```python
from build123d import *

# Parameters (mm, degrees)
SKETCH1_W           = 200
SKETCH1_H           = 150
BOSS_EXTRUDE1_DEPTH = 150
SKETCH2_R           = 14.834241456
CUT_EXTRUDE1_DEPTH  = 5
LPATTERN1_COUNT     = 3
LPATTERN1_PITCH     = 50
SKETCH3_W           = 17.49362466
SKETCH3_H           = 150
BOSS_EXTRUDE2_DEPTH = 50
SKETCH4_R           = 20.657727603
BOSS_EXTRUDE3_DEPTH = 30
SKETCH5_R           = 10
BOSS_EXTRUDE4_DEPTH = 60
SKETCH6_W           = 19.92759369
SKETCH6_H           = 8.419652836
SKETCH6_W_2         = 21.376212584
SKETCH6_H_2         = 8.0068992
CUT_EXTRUDE2_DEPTH  = 15


with BuildPart() as part:
    # Sketch1 → Boss-Extrude1 (new body)
    with BuildSketch(Plane.XY):
        Rectangle(SKETCH1_W, SKETCH1_H)
    extrude(amount=BOSS_EXTRUDE1_DEPTH)

    # Sketch2 → Cut-Extrude1 (cut)
    with BuildSketch(Plane(origin=(0, 0, 0), x_dir=(-1, 0, 0), z_dir=(0, 0, -1))):
        with Locations((80.018238541, 54.109118562)):
            Circle(SKETCH2_R)
    cut_extrude1 = extrude(amount=-CUT_EXTRUDE1_DEPTH, mode=Mode.SUBTRACT)

    # LPattern1: Cut-Extrude1 ×3
    with Locations(*[(0, -i * LPATTERN1_PITCH, 0) for i in range(1, LPATTERN1_COUNT)]):
        add(cut_extrude1, mode=Mode.SUBTRACT)

    # Sketch3 → Boss-Extrude2 (add)
    with BuildSketch(Plane(origin=(100, 0, 0), x_dir=(0, 0, -1), z_dir=(1, 0, 0))):
        with Locations((-125.713599326, 0)):
            Rectangle(SKETCH3_W, SKETCH3_H)
    extrude(amount=BOSS_EXTRUDE2_DEPTH)

    # Sketch4 → Boss-Extrude3 (add)
    with BuildSketch(Plane(origin=(0, 0, 116.966786996), x_dir=(-1, 0, 0), z_dir=(0, 0, -1))):
        with Locations(Location((-127.668059081, 0, 0), (0, 0, 180))):
            Circle(SKETCH4_R)
    extrude(amount=BOSS_EXTRUDE3_DEPTH)

    # Sketch5 → Boss-Extrude4 (add)
    with BuildSketch(Plane.XY.offset(150)):
        with Locations(Location((0, 0, 0), (0, 0, 180))):
            Circle(SKETCH5_R)
    extrude(amount=BOSS_EXTRUDE4_DEPTH)

    # Sketch6 → Cut-Extrude2 (cut)
    with BuildSketch(Plane.XY.offset(210)):
        with Locations((0.233720093, 6.517553958)):
            Rectangle(SKETCH6_W, SKETCH6_H)
        with Locations((-0.888741557, -5.9965504)):
            Rectangle(SKETCH6_W_2, SKETCH6_H_2)
    extrude(amount=-CUT_EXTRUDE2_DEPTH, mode=Mode.SUBTRACT)


solid = part.part
```
Build history of the part. All positions in model axes, mm. A direction names the side the tool comes from. Round coordinates to 2 decimals unless told otherwise and drop trailing zeros. Write each loop counter-clockwise with the first axis right and the second up, starting at its lowest first coordinate (ties: lowest second). Pieces come first, ordered by that corner, then holes.
1) Band-saw the part on A-A, the plane z = 97.5. List the corners of the cut face in (x, y).
2) Drill centre lines: probe 1 along X at (y, z) = (-32.5, 107.5); probe 2 along Z at (x, y) = (29, 11); probe 3 along Z at (x, y) = (102.5, 1). Where is each one in solid material? Low to high.
3) Pin check, flat tips, straight feed: pin 1 (12 mm diameter, centred on x = 4, z = 202, fed in from +Y); pin 2 (2.5 mm diameter, centred on x = 4.5, y = 5, fed in from +Z); pin 3 (9 mm diameter, centred on x = -75, y = -45.5, fed in from -Z); pin 4 (17 mm diameter, centred on y = 35, z = 140, fed in from +X). Stop position of each tip, or through.
4) Band-saw the part on C-C, the plane y = -42. List the corners of the cut face in (x, z), and give its area (3 significant figures).
5) Band-saw the part on B-B, the plane x = 0. List the corners of the cut face in (y, z).
6) Mould opens along X. For faces 6 (the flat face through (100, -1, 142)), 7 (the cylindrical face through (10, 0, 173)), 8 (the flat face through (0, 5, 195)), 9 (the cylindrical face through (-86.863, 40.949, 2.465)) say: +X half, -X half, draft (parallel to the pull), parting line (faces both ways), or undercut.
7) Band-saw the part on D-D, the plane z = 189.5. List the corners of the cut face in (x, y).
8) 3-axis set-ups, long thin cutter, end or side, ignore diameter. For faces 1 (the flat face through (-80, 4, 5)), 2 (the flat face through (125, -1, 134.46)), 3 (the flat face through (-1, 1, 0)), 4 (the flat face through (0, 2.308, 203)), 5 (the flat face through (0, -5, 195)): which of +Z, -Z, +X, -X, +Y, -Y reach the whole face in a straight line?
Ans:
1. outline: (-100, -75) - (100, -75) - (100, 75) - (-100, 75) - close; circle Ø41.32 at (127.67, 0)
2. probe 1: x = -100 to 100
2. probe 2: z = 0 to 150
2. probe 3: z = 116.97 to 134.46
3. pin 1: stops at y = 2.31
3. pin 2: stops at z = 195
3. pin 3: stops at z = 5
3. pin 4: stops at x = 150
4. outline: (-100, 0) - (-94.33, 0) - (-94.33, 5) - (-65.7, 5) - (-65.7, 0) - (100, 0) - (100, 116.97) - (150, 116.97) - (150, 134.46) - (100, 134.46) - (100, 150) - (-100, 150) - close
4. area: 30,700 mm2
5. outline: (-75, 0) - (75, 0) - (75, 150) - (10, 150) - (10, 195) - (2.31, 195) - (2.31, 210) - (-1.99, 210) - (-1.99, 195) - (-10, 195) - (-10, 150) - (-75, 150) - close
6. face 6: +X half
6. face 7: parting line
6. face 8: draft
6. face 9: undercut
7. outline: circle Ø20 at (0, 0)
8. face 1: -Z
8. face 2: +Z, +X, +Y, -Y
8. face 3: -Z, +X, -X, +Y, -Y
8. face 4: +Z, +X, -X, +Y
8. face 5: +Z, +X, -X, -Y
